Check sheet for the modelled part. Datum: model origin and axes. Units: mm. A direction names the side the tool comes from. Round coordinates to 2 decimals unless told otherwise and drop trailing zeros. Order: outer loops, then holes, each group sorted by start corner. A loop starts at its lowest first (then second) coordinate and runs counter-clockwise, first axis right, second up. Notation, with made-up numbers: (-21.75, 61) -> (1.25, 61) arc R7 ccw to (1.25, 66) -> close; hole circle Ø1 at (86.5, -15.5). An arc over 180 degrees is marked (long way). Answer in a Markdown table with one row per item. Add a question column.
1. Material ranges on L1, parallel to X at y = 16.5, z = 706.5 (3 decimals); L2, parallel to Y at x = 12, z = 521.5; L3, parallel to X at y = 22.5, z = 88.5, recorded low to high. Write a range as from..to.
2. Depth check by flat-ended pin: P1, Ø2.5, axis at x = 15, z = 566.5, coming from the -Y side; P2, Ø1, axis at x = 6.5, z = 449, coming from the +Y side. Enter the tip coordinate at first touch or a pass-through.
3. Sectioned sample at A-A, the plane y = 8.5. Record the boundary of the cut face in (x, z) (3 decimals).
4. Draft check along X on faces 1 (the flat face through (15, 29, 0)), 2 (the flat face through (28.702, 11, 375)), 3 (the flat face through (25.527, 9, 375)). Enter one of: +X half, -X half, draft (parallel to the pull), parting line (faces both ways), or undercut.
5. Access from +Z, -Z, +X, -X, +Y, -Y to the whole of each face (thin tool, end or side, straight path). Record for faces 4 (the flat face through (3.175, 9, 375)), 5 (the flat face through (14, 29, 760)).
6. Sectioned sample at B-B, the plane z = 539. Record the boundary of the cut face in (x, y) (3 decimals), then the cut area to 3 significant figures.
```python
from build123d import *

# Parameters (mm, degrees)
BOSS_EXTRUDE1_DEPTH = 825
SKETCH3_W           = 65
SKETCH3_H           = 21.75
CUT_EXTRUDE2_DEPTH  = 825


with BuildPart() as part:
    # Sketch1 → Boss-Extrude1 (new body)
    with BuildSketch(Plane.XY):
        with BuildLine():
            Line((3.175, 0), (3.175, 18.575))
            ThreePointArc((3.175, 18.575), (6.103932188, 25.646067812), (13.175, 28.575))
            Line((13.175, 28.575), (15.527, 28.575))
            ThreePointArc((15.527, 28.575), (22.598067812, 25.646067812), (25.527, 18.575))
            Line((25.527, 18.575), (25.527, 0))
            Line((25.527, 0), (28.702, 0))
            Line((28.702, 0), (28.702, 21.75))
            ThreePointArc((28.702, 21.75), (25.773067812, 28.821067812), (18.702, 31.75))
            Line((18.702, 31.75), (10, 31.75))
            ThreePointArc((10, 31.75), (2.928932188, 28.821067812), (0, 21.75))
            Line((0, 21.75), (0, 0))
            Line((0, 0), (3.175, 0))
        make_face()
    extrude(amount=BOSS_EXTRUDE1_DEPTH)

    # Sketch3 → Cut-Extrude2 (cut)
    with BuildSketch(Plane(origin=(28.702, 0, 0), x_dir=(0, 0, -1), z_dir=(1, 0, 0))):
        Polygon((-825, 21.75), (-760, 21.75), (-760, 58.136059774), (-855.704535521, 58.136059774), (-855.704535521, 0), (-825, 0), align=None)
        with Locations((-792.5, 10.875)):
            Rectangle(SKETCH3_W, SKETCH3_H)
    extrude(amount=-CUT_EXTRUDE2_DEPTH, mode=Mode.SUBTRACT)


solid = part.part
```
Answer key:
| question | item | result |
|---|---|---|
| 1 | L1 | x = 0..3.175, 25.527..28.702 |
| 1 | L2 | y = 28.51..31.75 |
| 1 | L3 | x = 0.03..3.98, 24.72..28.67 |
| 2 | P1 | stops at y = 28.55 |
| 2 | P2 | stops at y = 31.29 |
| 3 | outline | (0, 0) -> (3.175, 0) -> (3.175, 760) -> (0, 760) -> close; (25.527, 0) -> (28.702, 0) -> (28.702, 760) -> (25.527, 760) -> close |
| 4 | face 1 | draft |
| 4 | face 2 | +X half |
| 4 | face 3 | undercut |
| 5 | face 4 | +Z, -Z, -Y |
| 5 | face 5 | +Z, +X, -X, +Y, -Y |
| 6 | outline | (0, 0) -> (3.175, 0) -> (3.175, 18.575) arc R10 cw to (13.175, 28.575) -> (15.527, 28.575) arc R10 cw to (25.527, 18.575) -> (25.527, 0) -> (28.702, 0) -> (28.702, 21.75) arc R10 ccw to (18.702, 31.75) -> (10, 31.75) arc R10 ccw to (0, 21.75) -> close |
| 6 | area | 273 mm² |
